Geometry: final body of the model. Coordinates: model frame, mm. Face numbers are marked on the shaded views. A direction names the side the tool comes from. Coordinates: 2 decimals unless noted, no trailing zeros. Loops run counter-clockwise (first coordinate to the right, second up) from the corner with the lowest first, then second, coordinate; pieces in that order, holes last. Notation, with made-up numbers: (-3, -24) - (50, -24) arc R16 ccw to (50, -8) - close; hole circle Ø11 at (49, 87.25). An arc over 180 degrees is marked (long way). Write each question's results on one line, items separated by ' | '. Start each with the question number.
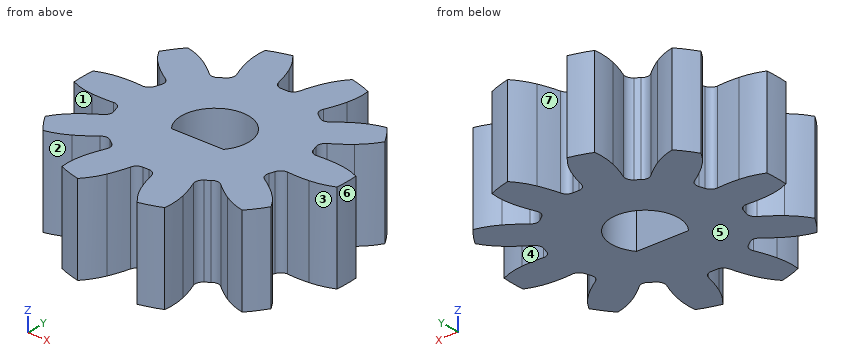
from build123d import *

# Parameters (mm, degrees)
SKETCH1_R                = 5.926666667
BLANK_DISK_DEPTH         = 2
GEAR_TOOTH_CUT_DEPTH     = 10.287128516
GEAR_START               = -2.000000064
GEAR_TEETH_REVOLVE_DEPTH = 4.000000128
SKETCH4_R                = 0.75
HUB_EXTRUDE_DEPTH        = 0.635
HEX_BORE_CUT_DEPTH       = 10.19015236
HEX_BORE_CUT_DEPTH_BACK  = 10.19015236


# Read off the part's stored shape, not the designer's step: GEAR TEETH REVOLVE
with BuildPart() as part:
    # Sketch1 → BLANK DISK (new, symmetric)
    with BuildSketch(Plane.XY):
        Circle(SKETCH1_R)
    extrude(amount=BLANK_DISK_DEPTH, both=True)

    # Sketch2 → GEAR TOOTH CUT (cut, through all)
    with BuildSketch(Plane.XY.offset(2.000000064)):
        with BuildLine():
            ThreePointArc((-5.077291995, -3.057201951), (-5.636594953, -1.83144072), (-5.90459373, -0.511029022))
            ThreePointArc((-5.90459373, -0.511029022), (-5.402476049, -0.687662082), (-4.877561226, -0.775899444))
            ThreePointArc((-4.877561226, -0.775899444), (-4.39839721, -0.795349357), (-3.919215726, -0.776334691))
            ThreePointArc((-3.919215726, -0.776334691), (-3.694949803, -0.83665634), (-3.55944947, -1.025265898))
            ThreePointArc((-3.55944947, -1.025265898), (-3.522871846, -1.14465045), (-3.482291287, -1.26273437))
            ThreePointArc((-3.482291287, -1.26273437), (-3.481051441, -1.494967805), (-3.627030209, -1.675589246))
            ThreePointArc((-3.627030209, -1.675589246), (-4.025872713, -1.941861868), (-4.402092173, -2.239242719))
            ThreePointArc((-4.402092173, -2.239242719), (-4.774892565, -2.619165437), (-5.077291995, -3.057201951))
        make_face()
    extrude(amount=-GEAR_TOOTH_CUT_DEPTH, mode=Mode.SUBTRACT)

    # GEAR TEETH REVOLVE outline → GEAR TEETH REVOLVE (cut)
    with BuildSketch(Plane.XY.offset(GEAR_START)):
        with BuildLine():
            ThreePointArc((-4.476541349, -3.884064278), (-3.483607262, -4.794774052), (-2.310637289, -5.457685689))
            ThreePointArc((-2.310637289, -5.457685689), (-2.323462415, -4.92556078), (-2.245173532, -4.399070273))
            ThreePointArc((-2.245173532, -4.399070273), (-2.115601674, -3.937347861), (-1.949442431, -3.487495042))
            ThreePointArc((-1.949442431, -3.487495042), (-1.937509746, -3.25556506), (-2.07501619, -3.068413027))
            ThreePointArc((-2.07501619, -3.068413027), (-2.177254539, -2.996733783), (-2.277018938, -2.92164944))
            ThreePointArc((-2.277018938, -2.92164944), (-2.497502926, -2.848706199), (-2.714394044, -2.931725163))
            ThreePointArc((-2.714394044, -2.931725163), (-3.090883469, -3.22876416), (-3.489967672, -3.494674392))
            ThreePointArc((-3.489967672, -3.494674392), (-3.966497305, -3.731826058), (-4.476541349, -3.884064278))
        make_face()
        with BuildLine():
            ThreePointArc((-1.338602326, -5.773518994), (0, -5.926666665), (1.338602326, -5.773518994))
            ThreePointArc((1.338602326, -5.773518994), (1.015451407, -5.35055932), (0.769325087, -4.878602501))
            ThreePointArc((0.769325087, -4.878602501), (0.602757298, -4.428900796), (0.472766097, -3.967296268))
            ThreePointArc((0.472766097, -3.967296268), (0.346094819, -3.772647115), (0.124844564, -3.7020622))
            ThreePointArc((0.124844564, -3.7020622), (0, -3.704166667), (-0.124844564, -3.7020622))
            ThreePointArc((-0.124844564, -3.7020622), (-0.346094819, -3.772647115), (-0.472766097, -3.967296268))
            ThreePointArc((-0.472766097, -3.967296268), (-0.602757298, -4.428900796), (-0.769325087, -4.878602501))
            ThreePointArc((-0.769325087, -4.878602501), (-1.015451407, -5.35055932), (-1.338602326, -5.773518994))
        make_face()
        with BuildLine():
            ThreePointArc((2.310637289, -5.457685689), (3.483607261, -4.794774052), (4.476541349, -3.884064278))
            ThreePointArc((4.476541349, -3.884064278), (3.966497305, -3.731826058), (3.489967672, -3.494674392))
            ThreePointArc((3.489967672, -3.494674392), (3.090883469, -3.22876416), (2.714394044, -2.931725163))
            ThreePointArc((2.714394044, -2.931725163), (2.497502926, -2.848706199), (2.277018938, -2.92164944))
            ThreePointArc((2.277018938, -2.92164944), (2.177254539, -2.996733783), (2.07501619, -3.068413027))
            ThreePointArc((2.07501619, -3.068413027), (1.937509746, -3.25556506), (1.949442431, -3.487495042))
            ThreePointArc((1.949442431, -3.487495042), (2.115601674, -3.937347861), (2.245173532, -4.399070273))
            ThreePointArc((2.245173532, -4.399070273), (2.323462415, -4.92556078), (2.310637289, -5.457685689))
        make_face()
        with BuildLine():
            ThreePointArc((5.077291995, -3.057201951), (5.636594953, -1.831440719), (5.904593729, -0.511029022))
            ThreePointArc((5.904593729, -0.511029022), (5.402476049, -0.687662082), (4.877561226, -0.775899444))
            ThreePointArc((4.877561226, -0.775899444), (4.398397211, -0.795349357), (3.919215726, -0.776334691))
            ThreePointArc((3.919215726, -0.776334691), (3.694949803, -0.83665634), (3.55944947, -1.025265898))
            ThreePointArc((3.55944947, -1.025265898), (3.522871846, -1.14465045), (3.482291287, -1.26273437))
            ThreePointArc((3.482291287, -1.26273437), (3.481051441, -1.494967805), (3.627030209, -1.675589246))
            ThreePointArc((3.627030209, -1.675589246), (4.025872713, -1.941861868), (4.402092173, -2.239242719))
            ThreePointArc((4.402092173, -2.239242719), (4.774892565, -2.619165437), (5.077291995, -3.057201951))
        make_face()
        with BuildLine():
            ThreePointArc((5.90459373, 0.511029022), (5.636594953, 1.83144072), (5.077291995, 3.057201951))
            ThreePointArc((5.077291995, 3.057201951), (4.774892565, 2.619165437), (4.402092173, 2.239242719))
            ThreePointArc((4.402092173, 2.239242719), (4.025872713, 1.941861868), (3.627030209, 1.675589246))
            ThreePointArc((3.627030209, 1.675589246), (3.481051441, 1.494967805), (3.482291287, 1.26273437))
            ThreePointArc((3.482291287, 1.26273437), (3.522871846, 1.14465045), (3.55944947, 1.025265898))
            ThreePointArc((3.55944947, 1.025265898), (3.694949803, 0.83665634), (3.919215726, 0.776334691))
            ThreePointArc((3.919215726, 0.776334691), (4.398397211, 0.795349357), (4.877561226, 0.775899444))
            ThreePointArc((4.877561226, 0.775899444), (5.402476049, 0.687662082), (5.90459373, 0.511029022))
        make_face()
        with BuildLine():
            ThreePointArc((4.47654135, 3.884064279), (3.483607262, 4.794774054), (2.310637289, 5.457685691))
            ThreePointArc((2.310637289, 5.457685691), (2.323462415, 4.92556078), (2.245173532, 4.399070273))
            ThreePointArc((2.245173532, 4.399070273), (2.115601674, 3.937347861), (1.949442431, 3.487495042))
            ThreePointArc((1.949442431, 3.487495042), (1.937509746, 3.25556506), (2.07501619, 3.068413027))
            ThreePointArc((2.07501619, 3.068413027), (2.177254539, 2.996733783), (2.277018938, 2.92164944))
            ThreePointArc((2.277018938, 2.92164944), (2.497502926, 2.848706199), (2.714394044, 2.931725163))
            ThreePointArc((2.714394044, 2.931725163), (3.090883469, 3.22876416), (3.489967672, 3.494674392))
            ThreePointArc((3.489967672, 3.494674392), (3.966497305, 3.731826058), (4.47654135, 3.884064279))
        make_face()
        with BuildLine():
            ThreePointArc((1.338602326, 5.773518996), (0, 5.926666667), (-1.338602326, 5.773518996))
            ThreePointArc((-1.338602326, 5.773518996), (-1.015451407, 5.35055932), (-0.769325087, 4.878602501))
            ThreePointArc((-0.769325087, 4.878602501), (-0.602757298, 4.428900796), (-0.472766097, 3.967296268))
            ThreePointArc((-0.472766097, 3.967296268), (-0.346094819, 3.772647115), (-0.124844564, 3.7020622))
            ThreePointArc((-0.124844564, 3.7020622), (0, 3.704166667), (0.124844564, 3.7020622))
            ThreePointArc((0.124844564, 3.7020622), (0.346094819, 3.772647115), (0.472766097, 3.967296268))
            ThreePointArc((0.472766097, 3.967296268), (0.602757298, 4.428900796), (0.769325087, 4.878602501))
            ThreePointArc((0.769325087, 4.878602501), (1.015451407, 5.35055932), (1.338602326, 5.773518996))
        make_face()
        with BuildLine():
            ThreePointArc((-2.31063729, 5.457685691), (-3.483607262, 4.794774054), (-4.47654135, 3.884064279))
            ThreePointArc((-4.47654135, 3.884064279), (-3.966497305, 3.731826058), (-3.489967672, 3.494674392))
            ThreePointArc((-3.489967672, 3.494674392), (-3.090883469, 3.22876416), (-2.714394044, 2.931725163))
            ThreePointArc((-2.714394044, 2.931725163), (-2.497502926, 2.848706199), (-2.277018938, 2.92164944))
            ThreePointArc((-2.277018938, 2.92164944), (-2.177254539, 2.996733783), (-2.07501619, 3.068413027))
            ThreePointArc((-2.07501619, 3.068413027), (-1.937509746, 3.25556506), (-1.949442431, 3.487495042))
            ThreePointArc((-1.949442431, 3.487495042), (-2.115601674, 3.937347861), (-2.245173532, 4.399070273))
            ThreePointArc((-2.245173532, 4.399070273), (-2.323462415, 4.92556078), (-2.31063729, 5.457685691))
        make_face()
        with BuildLine():
            ThreePointArc((-3.55944947, 1.025265898), (-3.522871846, 1.14465045), (-3.482291287, 1.26273437))
            ThreePointArc((-3.482291287, 1.26273437), (-3.481051441, 1.494967805), (-3.627030209, 1.675589246))
            ThreePointArc((-3.627030209, 1.675589246), (-4.025872713, 1.941861868), (-4.402092173, 2.239242719))
            ThreePointArc((-4.402092173, 2.239242719), (-4.774892565, 2.619165437), (-5.077291995, 3.057201951))
            ThreePointArc((-5.077291995, 3.057201951), (-5.636594954, 1.83144072), (-5.90459373, 0.511029022))
            ThreePointArc((-5.90459373, 0.511029022), (-5.402476049, 0.687662082), (-4.877561226, 0.775899444))
            ThreePointArc((-4.877561226, 0.775899444), (-4.398397211, 0.795349357), (-3.919215726, 0.776334691))
            ThreePointArc((-3.919215726, 0.776334691), (-3.694949803, 0.83665634), (-3.55944947, 1.025265898))
        make_face()
    extrude(amount=GEAR_TEETH_REVOLVE_DEPTH, mode=Mode.SUBTRACT)

    # Sketch4 → Hub Extrude (add)
    with BuildSketch(Plane.XY.offset(2.000000064)):
        Circle(SKETCH4_R)
    extrude(amount=HUB_EXTRUDE_DEPTH)

    # Sketch3 → HEX BORE CUT (cut, two sides: drawn at the far end of the back side and taken through both)
    with BuildSketch(Plane.XY.offset(2.000000064).offset(-HEX_BORE_CUT_DEPTH_BACK)):
        with BuildLine():
            Line((-1.168931136, -0.94), (1.168931136, -0.94))
            ThreePointArc((1.168931136, -0.94), (0, 1.5), (-1.168931136, -0.94))
        make_face()
    extrude(amount=HEX_BORE_CUT_DEPTH + HEX_BORE_CUT_DEPTH_BACK, mode=Mode.SUBTRACT)


solid = part.part
1) Section query B-B on x = 1. Output: boundary loops of the cut face in (y, z), and give its area (3 significant figures).
2) Section query C-C on x = -4.25. Output: boundary loops of the cut face in (y, z).
3) Pull-direction query (Y, two-part tool) for the marked faces 4, 5, 6 and 7; classes: released by +Y, released by -Y, zero draft, split by the parting line, or undercut.
4) Material intervals for line 1 (Y direction, x = 0, z = -1.05); line 2 (Y direction, x = 4.75, z = 1.1); line 3 (Y direction, x = -4.25, z = -0.5), sorted ascending. Write a range as [from, to].
5) Access query for the marked faces 1, 2 and 3. Directions: +Z, -Z, +X, -X, +Y, -Y. A direction counts if a zero-diameter tool reaches every point of the face in a straight line with its end or side. Return the directions, or none.
6) Section query A-A on y = 0. Output: boundary loops of the cut face in (x, z), and give its area (3 significant figures).
7) Pin query (flat end, axial travel): pin 1 Ø0.7 at (x, z) = (0, 0) entering from +Y; pin 2 Ø2 at (x, z) = (-4.5, -1) entering from +Y; pin 3 Ø1.8 at (x, y) = (0, 0) entering from +Z; pin 4 Ø1.5 at (x, z) = (1.5, 1) entering from -Y. Return the tip coordinate at first contact, or that it passes through.
Returned:
1) outline: (-5.33, -2) - (-0.94, -2) - (-0.94, 2) - (-5.33, 2) - close; (1.12, -2) - (5.33, -2) - (5.33, 2) - (1.12, 2) - close | area: 34.4 mm²
2) outline: (-3.83, -2) - (-2.11, -2) - (-2.11, 2) - (-3.83, 2) - close; (-0.79, -2) - (0.79, -2) - (0.79, 2) - (-0.79, 2) - close; (2.11, -2) - (3.83, -2) - (3.83, 2) - (2.11, 2) - close
3) face 4: undercut | face 5: zero draft | face 6: split by the parting line | face 7: released by +Y
4) line 1: y = [-3.7, -0.94], [1.5, 3.7] | line 2: y = [-3.54, -2.59], [-0.78, 0.78], [2.59, 3.54] | line 3: y = [-3.83, -2.11], [-0.79, 0.79], [2.11, 3.83]
5) face 1: +Z, -Z, -X | face 2: +Z, -Z, -Y | face 3: +Z, -Z, +X
6) outline: (-5.93, -2) - (-1.5, -2) - (-1.5, 2) - (-5.93, 2) - close; (1.5, -2) - (5.93, -2) - (5.93, 2) - (1.5, 2) - close | area: 35.4 mm²
7) pin 1: stops at y = 3.78 | pin 2: stops at y = 3.88 | pin 3: passes through | pin 4: stops at y = -5.77
